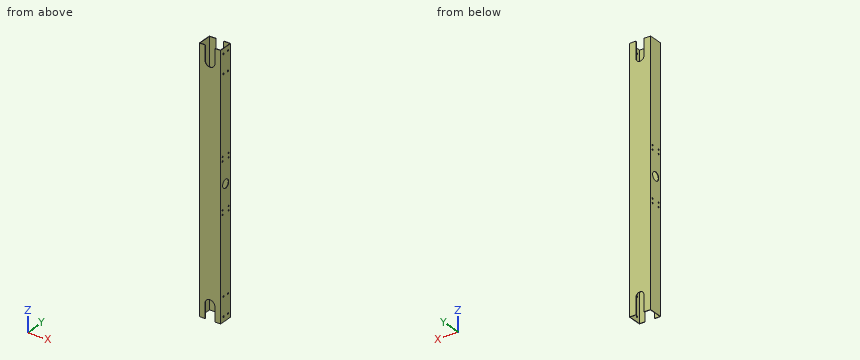
from build123d import *

# Parameters (mm, degrees)
SKETCH1_W           = 75
SKETCH1_H           = 50
SKETCH1_W_2         = 72
SKETCH1_H_2         = 47
BOSS_EXTRUDE1_DEPTH = 900
SKETCH2_R           = 15
CUT_EXTRUDE1_DEPTH  = 59
CUT_EXTRUDE2_DEPTH  = 10
CUT_EXTRUDE3_DEPTH  = 10
SKETCH5_R           = 3
CUT_EXTRUDE4_DEPTH  = 55
SKETCH7_R           = 2.5
CUT_EXTRUDE6_DEPTH  = 904.46554998
SKETCH8_R           = 15
CUT_EXTRUDE7_DEPTH  = 97


with BuildPart() as part:
    # Sketch1 → Boss-Extrude1 (new body)
    with BuildSketch(Plane.XY):
        Rectangle(SKETCH1_W, SKETCH1_H)
        Rectangle(SKETCH1_W_2, SKETCH1_H_2, mode=Mode.SUBTRACT)
    extrude(amount=BOSS_EXTRUDE1_DEPTH)

    # Sketch2 → Cut-Extrude1 (cut)
    with BuildSketch(Plane(origin=(37.5, 0, 0), x_dir=(0, 0, -1), z_dir=(1, 0, 0))):
        with Locations(Location((-450, 0, 0), (0, 0, 90))):
            Circle(SKETCH2_R)
    extrude(amount=-CUT_EXTRUDE1_DEPTH, mode=Mode.SUBTRACT)

    # Sketch3 → Cut-Extrude2 (cut)
    with BuildSketch(Plane(origin=(0, 25, 0), x_dir=(1, 0, 0), z_dir=(0, 1, 0))):
        with BuildLine():
            Line((14, -843), (14, -913.98611775))
            ThreePointArc((14, -913.98611775), (0, -927.98611775), (-14, -913.98611775))
            Line((-14, -913.98611775), (-14, -843))
            ThreePointArc((-14, -843), (0, -829), (14, -843))
        make_face()
    cut_extrude2 = extrude(amount=-CUT_EXTRUDE2_DEPTH, mode=Mode.SUBTRACT)

    # Sketch4 → Cut-Extrude3 (cut)
    with BuildSketch(Plane.XZ.offset(25)):
        with BuildLine():
            Line((-17.498938419, 850), (-17.498938419, 939.078503923))
            ThreePointArc((-17.498938419, 939.078503923), (0.001061581, 956.578503923), (17.501061581, 939.078503923))
            Line((17.501061581, 939.078503923), (17.501061581, 850))
            ThreePointArc((17.501061581, 850), (0.001061581, 832.5), (-17.498938419, 850))
        make_face()
    cut_extrude3 = extrude(amount=-CUT_EXTRUDE3_DEPTH, mode=Mode.SUBTRACT)

    # Sketch5 → Cut-Extrude4 (cut)
    with BuildSketch(Plane(origin=(37.5, 0, 0), x_dir=(0, 0, -1), z_dir=(1, 0, 0))):
        with Locations(Location((-882.5, 11, 0), (0, 0, 90))):
            Circle(SKETCH5_R)
        with Locations(Location((-882.5, -11, 0), (0, 0, 90))):
            Circle(SKETCH5_R)
        with Locations(Location((-816.5, -11, 0), (0, 0, 270))):
            Circle(SKETCH5_R)
        with Locations(Location((-816.5, 11, 0), (0, 0, 270))):
            Circle(SKETCH5_R)
    cut_extrude4 = extrude(amount=-CUT_EXTRUDE4_DEPTH, mode=Mode.SUBTRACT)

    # Mirror1: Cut-Extrude2, Cut-Extrude3, Cut-Extrude4 across plane
    add(cut_extrude2.mirror(Plane.XY.offset(450)), mode=Mode.SUBTRACT)
    add(cut_extrude3.mirror(Plane.XY.offset(450)), mode=Mode.SUBTRACT)
    add(cut_extrude4.mirror(Plane.XY.offset(450)), mode=Mode.SUBTRACT)

    # Sketch7 → Cut-Extrude6 (cut, through all)
    with BuildSketch(Plane.ZY.offset(37.5)):
        with Locations(Location((355, 15, 0), (0, 0, 270))):
            Circle(SKETCH7_R)
        with Locations(Location((370, 15, 0), (0, 0, 90))):
            Circle(SKETCH7_R)
        with Locations(Location((370, -15, 0), (0, 0, 270))):
            Circle(SKETCH7_R)
        with Locations(Location((355, -15, 0), (0, 0, 90))):
            Circle(SKETCH7_R)
        with Locations(Location((545, -15, 0), (0, 0, 270))):
            Circle(SKETCH7_R)
        with Locations(Location((530, -15, 0), (0, 0, 90))):
            Circle(SKETCH7_R)
        with Locations(Location((530, 15, 0), (0, 0, 270))):
            Circle(SKETCH7_R)
        with Locations(Location((545, 15, 0), (0, 0, 90))):
            Circle(SKETCH7_R)
    extrude(amount=-CUT_EXTRUDE6_DEPTH, mode=Mode.SUBTRACT)

    # Sketch8 → Cut-Extrude7 (cut)
    with BuildSketch(Plane(origin=(37.5, 0, 0), x_dir=(0, 0, -1), z_dir=(1, 0, 0))):
        with Locations(Location((-450, 0, 0), (0, 0, 90))):
            Circle(SKETCH8_R)
    extrude(amount=-CUT_EXTRUDE7_DEPTH, mode=Mode.SUBTRACT)


solid = part.part
Check sheet for the modelled part. Datum: model origin and axes. Units: mm. Give positions to 0.01 mm unless a question says otherwise; leave off trailing zeros. Loops run counter-clockwise (first coordinate to the right, second up) from the corner with the lowest first, then second, coordinate; pieces in that order, holes last. Notation, with made-up numbers: M 2.25,-13 L 30.25,-13 A18 ccw 30.25,16 Z; hole C 31,55 d11. An arc over 180 degrees is marked long. Answer as a JSON object with one key per item and string values. Group by question number.
Q1. Go/stop test with a flat-tipped pin: P1, Ø5.5, axis at y = 11, z = 882.5, coming from the +X side. Record where the tip stops, or that it passes through.
Q2. Material ranges on line 1 along Y through (x, z) = (37.05, 355); line 2 along X through (y, z) = (1, 87.5); line 3 along Y through (x, z) = (-21, 243.5), recorded low to high. Write a range as [from, to].
Q3. Cross-section at B-B on z = 756.5. Record the cut outline in (x, y).
Q4. Cross-section at A-A on x = 28.5. Record the cut outline in (y, z).
Q5. Cross-section at C-C on z = 450. Record the cut outline in (x, y).
Evaluation:
{
 "1": {"P1": "stops at x = -36"},
 "2": {"line 1": "y = [-25, -17.5], [-12.5, 12.5], [17.5, 25]", "line 2": "x = [-37.5, -36], [36, 37.5]", "line 3": "y = [-25, -23.5], [23.5, 25]"},
 "3": {"outline": "M -37.5,-25 L 37.5,-25 L 37.5,25 L -37.5,25 Z; hole M -36,-23.5 L 36,-23.5 L 36,23.5 L -36,23.5 Z"},
 "4": {"outline": "M -25,0 L -23.5,0 L -23.5,900 L -25,900 Z; M 23.5,0 L 25,0 L 25,900 L 23.5,900 Z"},
 "5": {"outline": "M -37.5,-25 L 37.5,-25 L 37.5,-15 L 36,-15 L 36,-23.5 L -36,-23.5 L -36,-15 L -37.5,-15 Z; M -37.5,15 L -36,15 L -36,23.5 L 36,23.5 L 36,15 L 37.5,15 L 37.5,25 L -37.5,25 Z"}
}
